For this review, use the dimensioned drawing (mm, ordinates from the lowest corner) and the shaded views. A direction names the side the tool comes from. Round coordinates to 2 decimals unless told otherwise and drop trailing zeros. Order: outer loops, then holes, each group sorted by start corner. A loop starts at its lowest first (then second) coordinate and runs counter-clockwise, first axis right, second up. Notation, with made-up numbers: (60, 14) - (68, 14) arc R19 ccw to (68, 50) - close; hole circle Ø9 at (41.25, 75.5). An arc over 180 degrees is marked (long way). Write item = value, one per line.
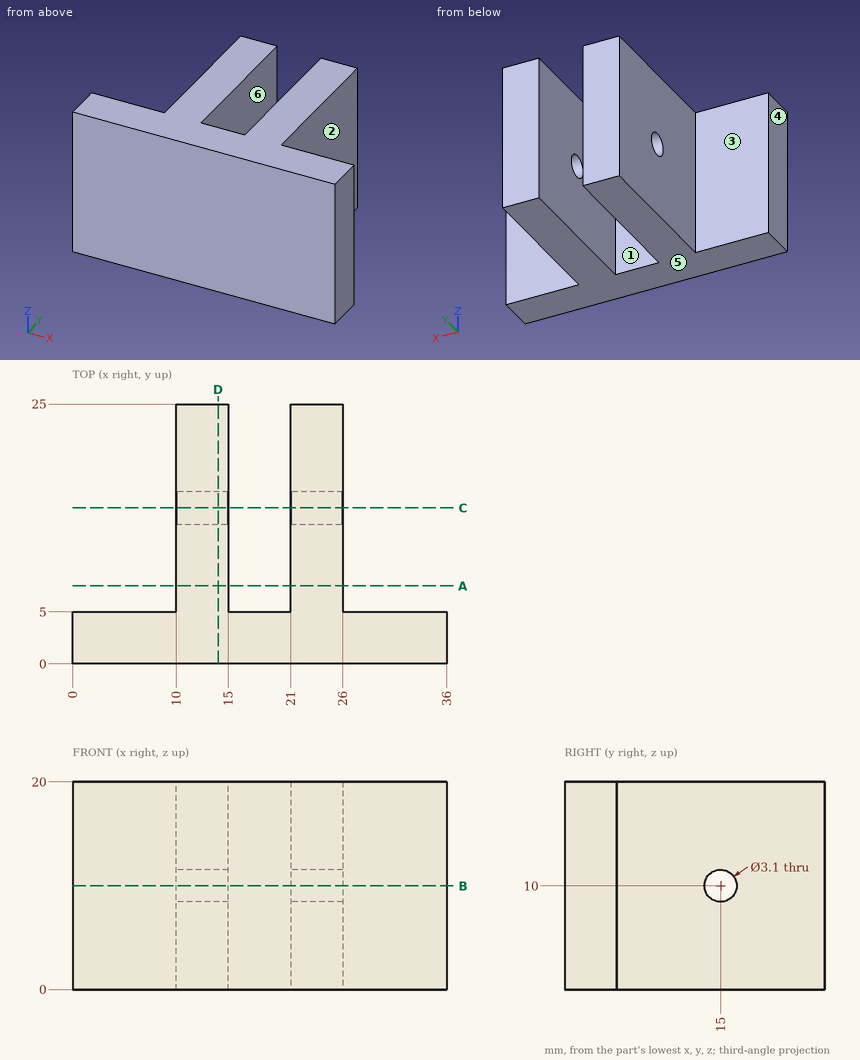
1) To check wall thickness, follow L1, parallel to X at y = 12, z = 14; L2, parallel to Z at x = 24.3, y = 15; L3, parallel to Y at x = 32, z = 9.25. State the ranges of each line that lie inside material, in increasing order. Write a range as from..to.
Findings:
L1 = 10..15, 21..26
L2 = 0..8.45, 11.55..20
L3 = 0..5
2) We need section B-B on z = 10. Write out the cut boundary in (x, y), and give its area (3 significant figures).
Findings:
outline = (0, 0) - (36, 0) - (36, 5) - (26, 5) - (26, 13.45) - (21, 13.45) - (21, 5) - (15, 5) - (15, 13.45) - (10, 13.45) - (10, 5) - (0, 5) - close; (10, 16.55) - (15, 16.55) - (15, 25) - (10, 25) - close; (21, 16.55) - (26, 16.55) - (26, 25) - (21, 25) - close
area = 349 mm^2
3) Clearance check with flat-ended pins moving along their axes: pin 1 Ø4 at (y, z) = (15, 10) entering from +X; pin 2 Ø5 at (y, z) = (11.5, 3) entering from -X; pin 3 Ø5 at (x, z) = (32.5, 10.5) entering from +Y; pin 4 Ø3 at (y, z) = (15, 10) entering from -X. State where each tip first meets the part, or that it passes through.
Findings:
pin_1 = 26
pin_2 = 10
pin_3 = 5
pin_4 = through
4) For the marked faces 1, 2 and 3, list the 3-axis set-ups (+Z, -Z, +X, -X, +Y, -Y) from which the entire face can be reached by the end or side of a thin tool; tool diameter is ignored.
Findings:
face_1 = +Z, -Z, +Y
face_2 = +Z, -Z, +X, +Y
face_3 = +Z, -Z, -X, +Y
5) We need section C-C on y = 15. Write out the cut boundary in (x, z).
Findings:
outline = (10, 0) - (15, 0) - (15, 8.45) - (10, 8.45) - close; (10, 11.55) - (15, 11.55) - (15, 20) - (10, 20) - close; (21, 0) - (26, 0) - (26, 8.45) - (21, 8.45) - close; (21, 11.55) - (26, 11.55) - (26, 20) - (21, 20) - close
6) We need section D-D on x = 14. Write out the cut boundary in (y, z), and give its area (3 significant figures).
Findings:
outline = (0, 0) - (25, 0) - (25, 20) - (0, 20) - close; hole circle Ø3.1 at (15, 10)
area = 492 mm^2
7) We need section A-A on y = 7.5. Write out the cut boundary in (x, z), and give its area (3 significant figures).
Findings:
outline = (10, 0) - (15, 0) - (15, 20) - (10, 20) - close; (21, 0) - (26, 0) - (26, 20) - (21, 20) - close
area = 200 mm^2
8) The part is to be moulded in two halves that separate along X. For the marked faces 4, 5 and 6, say which applies: released by +X, released by -X, zero draft, split by the parting line, or undercut.
Findings:
face_4 = released by -X
face_5 = zero draft
face_6 = undercut
